Source: CAD feature listing. Evaluate the final solid. Frame: model axes, mm. Face numbers are marked on the shaded views. A direction names the side the tool comes from. Give positions to 0.01 mm unless a question says otherwise; leave off trailing zeros. Loops run counter-clockwise (first coordinate to the right, second up) from the corner with the lowest first, then second, coordinate; pieces in that order, holes last.
from build123d import *

# Parameters (mm, degrees)
F0_R     = 11.25
F1_DEPTH = 7
F2_R     = 10


# Not quite as in the source:
# - a feature names something its author has since deleted; it is built from what else it names


with BuildPart() as f1:
    # F0 (on Top) → F1 (new body)
    with BuildSketch(Plane.XY):
        with BuildLine():
            ThreePointArc((2.7119035956, -16.0221121856), (12.4123110948, -10.4879470482), (16.25, 0))
            ThreePointArc((16.25, 0), (15.9933502519, 2.8766730299), (15.2315079728, 5.6624786864))
            ThreePointArc((15.2315079728, 5.6624786864), (14.0729128115, 8.125), (12.5196043772, 10.3596334992))
            ThreePointArc((12.5196043772, 10.3596334992), (0, 16.25), (-12.5196043772, 10.3596334992))
            ThreePointArc((-12.5196043772, 10.3596334992), (-14.0729128115, 8.125), (-15.2315079728, 5.6624786864))
            ThreePointArc((-15.2315079728, 5.6624786864), (-14.0729128115, -8.125), (-2.7119035956, -16.0221121856))
            ThreePointArc((-2.7119035956, -16.0221121856), (0, -16.25), (2.7119035956, -16.0221121856))
        make_face()
        Circle(F0_R, mode=Mode.SUBTRACT)
        with BuildLine():
            ThreePointArc((15.2315079728, 5.6624786864), (15.9933502519, 2.8766730299), (16.25, 0))
            ThreePointArc((16.25, 0), (12.4123110948, -10.4879470482), (2.7119035956, -16.0221121856))
            Line((2.7119035956, -16.0221121856), (15.101342571, -21.9861975129))
            ThreePointArc((15.101342571, -21.9861975129), (15.8049636191, -9.125), (26.5912768643, -2.0850475413))
            Line((26.5912768643, -2.0850475413), (15.2315079728, 5.6624786864))
        make_face()
        with BuildLine():
            ThreePointArc((-12.5196043772, 10.3596334992), (0, 16.25), (12.5196043772, 10.3596334992))
            Line((12.5196043772, 10.3596334992), (11.4899342932, 24.0712450542))
            ThreePointArc((11.4899342932, 24.0712450542), (0, 18.25), (-11.4899342932, 24.0712450542))
            Line((-11.4899342932, 24.0712450542), (-12.5196043772, 10.3596334992))
        make_face()
        with BuildLine():
            ThreePointArc((42.395825623, -16.25), (37.6566137131, -5.6383361387), (26.5912768643, -2.0850475413))
            ThreePointArc((26.5912768643, -2.0850475413), (15.8049636191, -9.125), (15.101342571, -21.9861975129))
            ThreePointArc((15.101342571, -21.9861975129), (31.0765777883, -30.1953645254), (42.395825623, -16.25))
        make_face()
        with Locations((28.145825623, -16.25)):
            Circle(F0_R, mode=Mode.SUBTRACT)
        with BuildLine():
            Line((-15.101342571, -21.9861975129), (-2.7119035956, -16.0221121856))
            ThreePointArc((-2.7119035956, -16.0221121856), (-14.0729128115, -8.125), (-15.2315079728, 5.6624786864))
            Line((-15.2315079728, 5.6624786864), (-26.5912768643, -2.0850475413))
            ThreePointArc((-26.5912768643, -2.0850475413), (-17.5341617617, -6.7392119099), (-13.895825623, -16.25))
            ThreePointArc((-13.895825623, -16.25), (-14.2004610976, -19.1807521653), (-15.101342571, -21.9861975129))
        make_face()
        with BuildLine():
            ThreePointArc((-11.4899342932, 24.0712450542), (0, 18.25), (11.4899342932, 24.0712450542))
            ThreePointArc((11.4899342932, 24.0712450542), (13.5424160267, 28.0654235647), (14.25, 32.5))
            ThreePointArc((14.25, 32.5), (-4.4345764353, 46.0424160267), (-11.4899342932, 24.0712450542))
        make_face()
        with Locations((0, 32.5)):
            Circle(F0_R, mode=Mode.SUBTRACT)
        with BuildLine():
            ThreePointArc((-26.5912768643, -2.0850475413), (-40.4866876269, -23.375), (-15.101342571, -21.9861975129))
            ThreePointArc((-15.101342571, -21.9861975129), (-14.2004610976, -19.1807521653), (-13.895825623, -16.25))
            ThreePointArc((-13.895825623, -16.25), (-17.5341617617, -6.7392119099), (-26.5912768643, -2.0850475413))
        make_face()
        with Locations((-28.145825623, -16.25)):
            Circle(F0_R, mode=Mode.SUBTRACT)
    extrude(amount=F1_DEPTH)

    # F2
    f2_edges = [f1.edges().sort_by_distance(p)[0] for p in [
        (-11.489934, 24.071245, 3.5),
        (-12.519604, 10.359633, 3.5),
        (-15.231508, 5.662479, 3.5),
        (-26.591277, -2.085048, 3.5),
        (2.711904, -16.022112, 3.5),
        (-2.711904, -16.022112, 3.5),
        (15.101343, -21.986198, 3.5),
        (-15.101343, -21.986198, 3.5),
        (26.591277, -2.085048, 3.5),
        (15.231508, 5.662479, 3.5),
        (12.519604, 10.359633, 3.5),
        (11.489934, 24.071245, 3.5),
    ]]
    fillet(f2_edges, radius=F2_R)


solid = f1.part
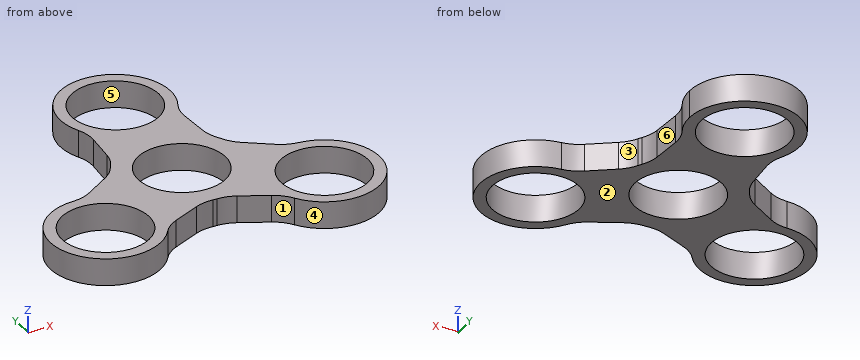
1) Pull-direction query (Y, two-part tool) for the marked faces 3, 4, 5 and 6; classes: released by +Y, released by -Y, zero draft, split by the parting line, or undercut.
Checks:
face 3: released by +Y
face 4: split by the parting line
face 5: undercut
face 6: undercut
2) Cut plane C-C (y = 31). Return loops of the section in (x, z).
Checks:
outline: (-14.17, 0) - (-11.15, 0) - (-11.15, 7) - (-14.17, 7) - close; (11.15, 0) - (14.17, 0) - (14.17, 7) - (11.15, 7) - close
3) Cut plane A-A (z = 5). Return loops of the section in (x, y).
Checks:
outline: (-29.01, -2.03) arc R14.25 ccw (long way) to (-16.26, -24.11) arc R10 cw to (-12.26, -20.62) - (-5.21, -17.23) arc R10 cw to (-0.54, -16.24) arc R16.25 ccw to (0.54, -16.24) arc R10 cw to (5.21, -17.23) - (12.26, -20.62) arc R10 cw to (16.26, -24.11) arc R14.25 ccw (long way) to (29.01, -2.03) arc R10 cw to (23.98, -0.31) - (17.52, 4.1) arc R10 cw to (14.34, 7.65) arc R16.25 ccw to (13.79, 8.59) arc R10 cw to (12.31, 13.13) - (11.73, 20.92) arc R10 cw to (12.75, 26.14) arc R14.25 ccw (long way) to (-12.75, 26.14) arc R10 cw to (-11.73, 20.92) - (-12.31, 13.13) arc R10 cw to (-13.79, 8.59) arc R16.25 ccw to (-14.34, 7.65) arc R10 cw to (-17.52, 4.1) - (-23.98, -0.31) arc R10 cw to start; hole circle Ø22.5 at (-28.15, -16.25); hole circle Ø22.5 at (0, 0); hole circle Ø22.5 at (0, 32.5); hole circle Ø22.5 at (28.15, -16.25)
4) Reachability of the marked faces 1 and 2 from +Z, -Z, +X, -X, +Y, -Y: full face, straight path, thin tool, end or side. Return the list, or none.
Checks:
face 1: +Z, -Z, -Y
face 2: -Z, +X, -X, +Y, -Y
5) Cut plane B-B (x = -25.5). Return loops of the section in (y, z), and give its area (3 significant figures).
Checks:
outline: (-30.25, 0) - (-27.18, 0) - (-27.18, 7) - (-30.25, 7) - close; (-5.32, 0) - (-1.16, 0) - (-1.16, 7) - (-5.32, 7) - close
area: 50.6 mm2
6) Cut plane D-D (y = -13.5). Return loops of the section in (x, z), and give its area (3 significant figures).
Checks:
outline: (-42.13, 0) - (-39.05, 0) - (-39.05, 7) - (-42.13, 7) - close; (-17.24, 0) - (17.24, 0) - (17.24, 7) - (-17.24, 7) - close; (39.05, 0) - (42.13, 0) - (42.13, 7) - (39.05, 7) - close
area: 284 mm2
7) Contact query for flat-ended pins moving along their axis: P1, Ø20, axis at x = -28.15, y = -16.25, coming from the -Z side; P2, Ø1.5, axis at y = 24, z = 4, coming from the -X side; P3, Ø2, axis at y = 22.5, z = 2.5, coming from the -X side; P4, Ø2, axis at x = 28, z = 3, coming from the +Y side. Output: stop coordinate, or through.
Checks:
P1: passes through
P2: stops at x = -12.18
P3: stops at x = -11.87
P4: stops at y = -1.7
8) Ray query, probe 1 along Y at (x, z) = (0, 4.75); probe 2 along Y at (x, z) = (-1.5, 3.5); probe 3 along X at (y, z) = (-10, 4.5). Return the intervals inside material, ascending.
Checks:
probe 1: y = -16.25 to -11.25, 11.25 to 21.25, 43.75 to 46.75
probe 2: y = -16.26 to -11.15, 11.15 to 21.35, 43.65 to 46.67
probe 3: x = -40.95 to -37.5, -18.79 to -5.15, 5.15 to 18.79, 37.5 to 40.95
